Check sheet for the modelled part. Datum: model origin and axes. Units: mm. A direction names the side the tool comes from. Round coordinates to 2 decimals unless told otherwise and drop trailing zeros. Loops run counter-clockwise (first coordinate to the right, second up) from the corner with the lowest first, then second, coordinate; pieces in that order, holes last. Notation, with made-up numbers: M -32.5,24.25 L -10.5,24.25 A15 ccw -10.5,34.25 Z; hole C -25.75,3.25 d7. An arc over 180 degrees is marked long. One line per question, with ' | ' between items. Start each with the question number.
(1) Section check C-C (z = 6.25). Record the boundary of the cut face in (x, y).
(2) Tool access check on faces 4 (the face through (747.75, 558, 6)), 5 (the face through (703, 554.143, 6)), 6 (the face through (703, 561.643, 6)), 7 (the face through (666.228, 572, -3)). Record the directions out of +Z, -Z, +X, -X, +Y, -Y that give a thin tool (end or side, any length) a straight path to the whole face; none if there is none.
(3) Thickness scan on probe 1 along X at (y, z) = (527, -1); probe 2 along X at (y, z) = (554.5, 4); probe 3 along Z at (x, y) = (701.5, 540). Record the ranges inside material, lowest first. Write a range as [from, to].
(4) Draft check along X on faces 1 (the face through (600.478, 546, -3)), 2 (the face through (667.528, 572, -3)), 3 (the face through (712, 547, 0)). Enter one of: +X half, -X half, draft (parallel to the pull), parting line (faces both ways), or undercut.
(5) Section check A-A (x = 715). Record the boundary of the cut face in (y, z).
(6) Section check B-B (y = 556.5). Record the boundary of the cut face in (x, z).
(7) Go/stop test with flat-tipped pins: P1, Ø2.5, axis at x = 806.48, y = 527.59, coming from the +Z side; P2, Ø9, axis at x = 693, z = 8, coming from the +Y side; P3, Ø10, axis at x = 653, y = 568, coming from the +Z side; P4, Ø5.5, axis at x = 684.5, z = 5, coming from the -Y side. Record where each tip stops, or that it passes through.
(8) Section check D-D (x = 643). Record the boundary of the cut face in (y, z), and give its area (3 significant figures).
```python
from build123d import *

# Parameters (mm, degrees)
BOSS_EXTRUDE1_DEPTH = 6.35
SKETCH2_R           = 2.20000068
CUT_EXTRUDE1_DEPTH  = 1004.989260418
SKETCH3_W           = 88.9999998
SKETCH3_H           = 7.4999977
BOSS_EXTRUDE2_DEPTH = 11.43


with BuildPart() as part:
    # 3DSketch1 → Boss-Extrude1 (new body)
    with BuildSketch(Plane(origin=(600.47776272, 523.59342576, 0), x_dir=(0.9797149309198314, 0.20039624281096213, 0), z_dir=(0, 0, 1))):
        with BuildLine():
            Line((0, 0), (9.017831215, 44.087173302))
            ThreePointArc((9.017831215, 44.087173302), (13.304365371, 50.427857212), (20.81894333, 51.880360433))
            Line((20.81894333, 51.880360433), (74.458631652, 40.908605623))
            ThreePointArc((74.458631652, 40.908605623), (75.092700365, 40.47995199), (75.237950761, 39.728493812))
            Line((75.237950761, 39.728493812), (73.073671595, 29.147573812))
            ThreePointArc((73.073671595, 29.147573812), (73.102720392, 28.99728113), (73.229534512, 28.911549561))
            Line((73.229534512, 28.911549561), (74.111278675, 28.731192794))
            ThreePointArc((74.111278675, 28.731192794), (74.261570989, 28.760243499), (74.347300947, 28.887058709))
            Line((74.347300947, 28.887058709), (76.511580113, 39.467978708))
            ThreePointArc((76.511580113, 39.467978708), (76.940233746, 40.102047422), (77.691691924, 40.247297817))
            Line((77.691691924, 40.247297817), (97.731759327, 36.148192979))
            ThreePointArc((97.731759327, 36.148192979), (98.36582804, 35.719539346), (98.511078436, 34.968081168))
            Line((98.511078436, 34.968081168), (96.34679927, 24.387161168))
            ThreePointArc((96.34679927, 24.387161168), (96.375848066, 24.236868486), (96.502662187, 24.151136917))
            Line((96.502662187, 24.151136917), (97.38440635, 23.97078015))
            ThreePointArc((97.38440635, 23.97078015), (97.534698663, 23.999830856), (97.620428621, 24.126646065))
            Line((97.620428621, 24.126646065), (99.784707787, 34.707566065))
            ThreePointArc((99.784707787, 34.707566065), (100.21336142, 35.341634778), (100.964819598, 35.486885174))
            Line((100.964819598, 35.486885174), (216.761930807, 11.801111606))
            ThreePointArc((216.761930807, 11.801111606), (223.102612928, 7.514576899), (224.555115449, 0))
            Line((224.555115449, 0), (215.537284234, -44.087173302))
            ThreePointArc((215.537284234, -44.087173302), (211.250750587, -50.427854723), (203.736175117, -51.880358453))
            Line((203.736175117, -51.880358453), (7.793187639, -11.801109626))
            ThreePointArc((7.793187639, -11.801109626), (1.45250443, -7.514576531), (0, 0))
        make_face()
    extrude(amount=-BOSS_EXTRUDE1_DEPTH)

    # Sketch2 → Cut-Extrude1 (cut, through all)
    with BuildSketch(Plane.XY):
        with Locations((806.4777622, 527.59342792)):
            Circle(SKETCH2_R)
        with Locations((806.47776474, 564.59342758)):
            Circle(SKETCH2_R)
        with Locations((628.49137192, 527.59342792)):
            Circle(SKETCH2_R)
        with Locations((628.43782872, 564.59342758)):
            Circle(SKETCH2_R)
    extrude(amount=-CUT_EXTRUDE1_DEPTH, mode=Mode.SUBTRACT)

    # Sketch3 → Boss-Extrude2 (add)
    with BuildSketch(Plane.XY):
        with Locations((703.25022672, 557.89342701)):
            Rectangle(SKETCH3_W, SKETCH3_H)
    extrude(amount=BOSS_EXTRUDE2_DEPTH)


solid = part.part
```
The answers:
1) outline: M 658.75,554.14 L 747.75,554.14 L 747.75,561.64 L 658.75,561.64 Z
2) face 4: +Z, +X, +Y, -Y | face 5: +Z, +X, -X, -Y | face 6: +Z, +X, -X, +Y | face 7: +Z, -Z, +Y
3) probe 1: [600.48, 626.37], [630.61, 804.36], [808.6, 820.48] | probe 2: [658.75, 747.75] | probe 3: [-6.35, 0]
4) face 1: -X half | face 2: undercut | face 3: draft
5) outline: M 513.59,-6.35 L 578.59,-6.35 L 578.59,0 L 561.64,0 L 561.64,11.43 L 554.14,11.43 L 554.14,0 L 513.59,0 Z
6) outline: M 600.48,-6.35 L 820.48,-6.35 L 820.48,0 L 747.75,0 L 747.75,11.43 L 658.75,11.43 L 658.75,0 L 600.48,0 Z
7) P1: through | P2: y = 561.64 | P3: z = 0 | P4: y = 554.14
8) outline: M 513.59,-6.35 L 578.59,-6.35 L 578.59,0 L 513.59,0 Z | area: 413 mm²
